Input: part model. Units: mm. Frame: model coordinates. Face numbers are marked on the shaded views. A direction names the side the tool comes from. Give positions to 0.01 mm unless a question says otherwise; leave off trailing zeros. Loops run counter-clockwise (first coordinate to the right, second up) from the corner with the lowest first, then second, coordinate; pieces in that order, holes last. Notation, with made-up numbers: (56, 78) -> (63, 78) arc R29 ccw to (63, 99) -> close; hole circle Ø1 at (14, -7.5). An arc over 180 degrees is marked (long way). Use CSV: the item, a comma, the result in double quotes.
Autodesk Inventor part; units mm, degrees
ref_plane "YZ Plane" through (0, 0, 0) normal (1, 0, 0) x (0, 1, 0)
ref_plane "XZ Plane" through (0, 0, 0) normal (0, 1, 0) x (-1, 0, 0)
ref_plane "XY Plane" through (0, 0, 0) normal (0, 0, 1) x (1, 0, 0)
ref_plane "Work Plane1" through (0, 0, 0) normal (0, 0, 1) x (1, 0, 0)
sketch "Sketch1" plane through (0, 0, 0) normal (0, 0, 1) x (1, 0, 0)
  line L0 (0, -789.9925) -> (25.4, -789.9925)
  line L1 (25.4, -789.9925) -> (25.4, -180.3925)
  line L2 (25.4, -180.3925) -> (0, -180.3925)
  line L3 (0, -180.3925) -> (0, -789.9925)
  point P0 (0, 0)
  dimension "d0" = 25.4
  dimension "d1" = 609.6
extrude "Extrusion1" add sketch "Sketch1" along normal blind 25.4
ref_plane "Work Plane2" through (0, 0, 12.7) normal (0, 0, 1) x (1, 0, 0)
sketch "Sketch3" plane through (0, 0, 12.7) normal (0, 0, 1) x (1, 0, 0)
  line L0 (0, -180.3925) -> (0, -789.9925)
  line L1 (0, -761.3575) -> (0, -456.5575)
  line L2 (0, -456.5575) -> (-457.2, -608.9575)
  line L3 (-457.2, -608.9575) -> (0, -761.3575)
  point P0 (0, 0)
  dimension "d8" = 304.8
  dimension "d9" = 457.2
extrude "Extrusion2" add sketch "Sketch3" along normal mid plane 2.54
properties part number "flag holder"
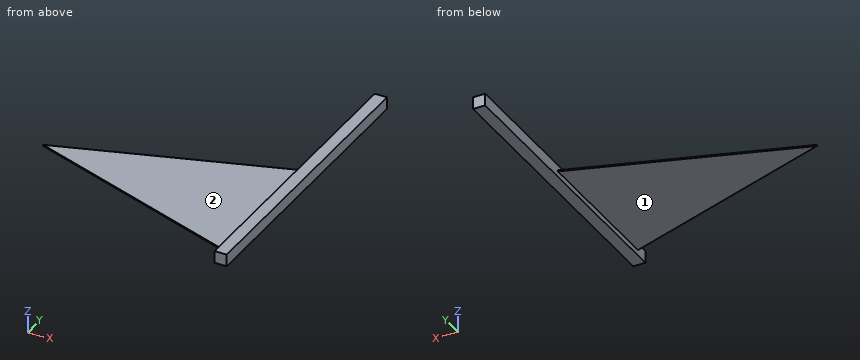
1) Ray query, line 1 (X direction, y = -468, z = 1.5); line 2 (Z direction, x = -36.5, y = -489.5). Return the intervals inside material, ascending.
From the geometry:
line 1,"x = 0 to 25.4"
line 2,"z = 11.43 to 13.97"
2) Section query D-D (y = -731.5). Return loops of the section in (x, z), then the cut area to 3 significant figures.
From the geometry:
outline,"(-89.57, 11.43) -> (0, 11.43) -> (0, 0) -> (25.4, 0) -> (25.4, 25.4) -> (0, 25.4) -> (0, 13.97) -> (-89.57, 13.97) -> close"
area,"873 mm^2"
3) Section query A-A (y = -338.5). Return loops of the section in (x, z), then the cut area to 3 significant figures.
From the geometry:
outline,"(0, 0) -> (25.4, 0) -> (25.4, 25.4) -> (0, 25.4) -> close"
area,"645 mm^2"
4) Section query B-B (z = 18.25). Return loops of the section in (x, y), then the cut area to 3 significant figures.
From the geometry:
outline,"(0, -789.99) -> (25.4, -789.99) -> (25.4, -180.39) -> (0, -180.39) -> close"
area,"15,500 mm^2"
5) Contact query for flat-ended pins moving along their axis: pin 1 (1 mm diameter, centred on y = -528.5, z = 16.5, fed in from -X); pin 2 (12 mm diameter, centred on x = -152.5, y = -673.5, fed in from +Z); pin 3 (3 mm diameter, centred on x = -30, z = 12.5, fed in from -Y). Output: stop coordinate, or through.
From the geometry:
pin 1,"stops at x = 0"
pin 2,"stops at z = 13.97"
pin 3,"stops at y = -751.86"
6) Reachability of the marked faces 1 and 2 from +Z, -Z, +X, -X, +Y, -Y: full face, straight path, thin tool, end or side. Return the list, or none.
From the geometry:
face 1,"-Z, -X, +Y, -Y"
face 2,"+Z, -X, +Y, -Y"
7) Section query C-C (y = -646). Return loops of the section in (x, z), then the cut area to 3 significant figures.
From the geometry:
outline,"(-346.07, 11.43) -> (0, 11.43) -> (0, 0) -> (25.4, 0) -> (25.4, 25.4) -> (0, 25.4) -> (0, 13.97) -> (-346.07, 13.97) -> close"
area,"1,520 mm^2"
